Geometry: see drawing. Coordinates: mm, zero at the bounding-box minimum. A direction names the side the tool comes from. Give positions to 0.01 mm unless a question says otherwise; leave off trailing zeros. Write each loop counter-clockwise with the first axis right and the second up, starting at its lowest first coordinate (ties: lowest second). Pieces come first, ordered by that corner, then holes.
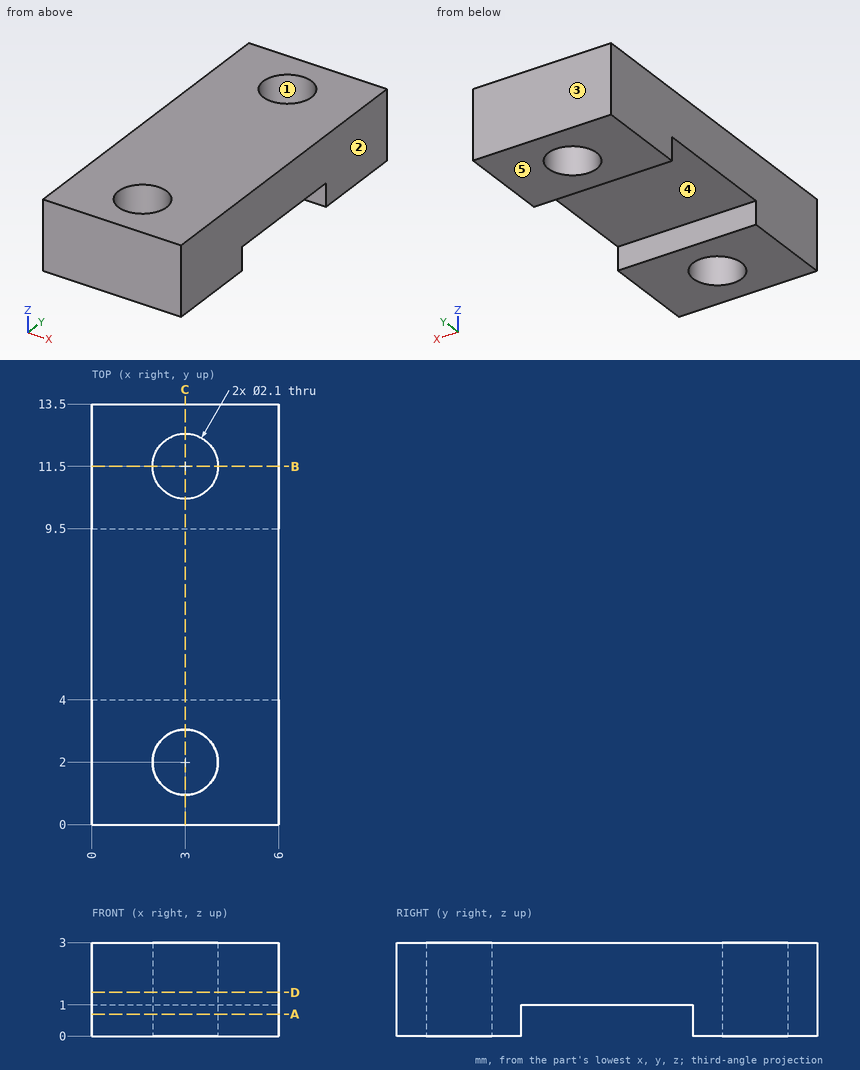
Q1. Section A-A, the plane z = 0.7. Return the cut outline in (x, y), then the cut area to 3 significant figures.
Q2. Section B-B, the plane y = 11.5. Return the cut outline in (x, z).
Q3. Mould query, pull axis X, two halves, no side actions, for the marked faces 1, 2 and 3. Classes: +X half, -X half, draft (parallel to the pull), parting line (faces both ways), or undercut.
Q4. Section C-C, the plane x = 3. Return the cut outline in (y, z), then the cut area to 3 significant figures.
Q5. Material intervals for line 1 along Y through (x, z) = (3, 2.05); line 2 along X through (y, z) = (11.5, 1.45); line 3 along X through (y, z) = (11, 2.3), sorted ascending.
Q6. Section D-D, the plane z = 1.4. Return the cut outline in (x, y).
Q7. Pin query (flat end, axial travel): pin 1 (1 mm diameter, centred on x = 3.5, y = 7, fed in from -Z). Return the tip coordinate at first contact, or that it passes through.
Q8. Access query for the marked faces 4 and 5. Directions: +Z, -Z, +X, -X, +Y, -Y. A direction counts if a zero-diameter tool reaches every point of the face in a straight line with its end or side. Return the directions, or none.
Solutions:
1. outline: (0, 0) - (6, 0) - (6, 4) - (0, 4) - close; (0, 9.5) - (6, 9.5) - (6, 13.5) - (0, 13.5) - close; hole circle Ø2.1 at (3, 2); hole circle Ø2.1 at (3, 11.5)
1. area: 41.1 mm2
2. outline: (0, 0) - (1.95, 0) - (1.95, 3) - (0, 3) - close; (4.05, 0) - (6, 0) - (6, 3) - (4.05, 3) - close
3. face 1: undercut
3. face 2: +X half
3. face 3: draft
4. outline: (0, 0) - (0.95, 0) - (0.95, 3) - (0, 3) - close; (3.05, 0) - (4, 0) - (4, 1) - (9.5, 1) - (9.5, 0) - (10.45, 0) - (10.45, 3) - (3.05, 3) - close; (12.55, 0) - (13.5, 0) - (13.5, 3) - (12.55, 3) - close
4. area: 22.4 mm2
5. line 1: y = 0 to 0.95, 3.05 to 10.45, 12.55 to 13.5
5. line 2: x = 0 to 1.95, 4.05 to 6
5. line 3: x = 0 to 2.08, 3.92 to 6
6. outline: (0, 0) - (6, 0) - (6, 13.5) - (0, 13.5) - close; hole circle Ø2.1 at (3, 2); hole circle Ø2.1 at (3, 11.5)
7. pin 1: stops at z = 1
8. face 4: -Z, +X, -X
8. face 5: -Z, +X, -X, +Y, -Y
